```python
from build123d import *

# Parameters (mm, degrees)
F1_DEPTH = 3


with BuildPart() as f1:
    # F0 (on Top) → F1 (new body)
    with BuildSketch(Plane.XY):
        Polygon((-1.428907, -2.407704), (2.857814, 2.211777), (2.208733, 3.138307), (1.428907, 2.103039), (-2.857814, -2.516442), (-2.215881, -3.284665), align=None)
        Polygon((-2.857814, -4), (-2.215881, -3.284665), (-2.857814, -2.516442), align=None)
        Polygon((0.730746, -4), (-1.618143, -4), (-2.857814, -4), (-2.857814, -5), (2.005268, -5), (1.983487, -4), align=None)
        Polygon((1.633301, -2.505144), (1.983487, -4), (1.983487, -1.925149), align=None)
        Polygon((1.633301, -2.505144), (0.730746, -4), (1.983487, -4), align=None)
        Polygon((1.605074, 4), (2.857814, 4), (2.857814, 5), (-1.996555, 5), (-1.996555, 4), (-0.743815, 4), align=None)
        Polygon((-1.747311, 3.100817), (-1.996555, 4), (-1.996555, 2.877482), align=None)
        Polygon((-1.296617, 1.474879), (-1.747311, 3.100817), (-1.996555, 2.877482), (-1.996555, 1.474879), align=None)
        Polygon((-1.747311, 3.100817), (-0.743815, 4), (-1.996555, 4), align=None)
        Polygon((1.257835, -0.902368), (1.633301, -2.505144), (1.983487, -1.925149), (1.983487, -0.902368), align=None)
        Polygon((2.208733, 3.138307), (2.857814, 2.211777), (2.857814, 4), align=None)
        Polygon((-1.618143, -4), (-2.215881, -3.284665), (-2.857814, -4), align=None)
        Polygon((2.208733, 3.138307), (2.857814, 4), (1.605074, 4), align=None)
    extrude(amount=F1_DEPTH)


solid = f1.part
```
Geometry check sheet. Reference: the model listing, model coordinates, mm. A direction names the side the tool comes from. Give positions to 0.01 mm unless a question says otherwise; leave off trailing zeros. Loops run counter-clockwise (first coordinate to the right, second up) from the corner with the lowest first, then second, coordinate; pieces in that order, holes last. Notation, with made-up numbers: M -22,11.5 L 14,11.5 A10 cw 14,25.5 Z; hole C 41,76 d5. An arc over 180 degrees is marked long. Write item = value, one per line. Start each with the question number.
1. Tool access check on faces 1 (the face through (0, 5, 1)), 2 (the face through (1.983, -2, 1)), 3 (the face through (-1.52, 2.28, 1.48)). Record the directions out of +Z, -Z, +X, -X, +Y, -Y that give a thin tool (end or side, any length) a straight path to the whole face; none if there is none.
2. Draft check along X on faces 4 (the face through (-1.997, 3, 1)), 5 (the face through (0.684, -0.13, 1.479)), 6 (the face through (0, -5, 1)). Enter one of: +X half, -X half, draft (parallel to the pull), parting line (faces both ways), or undercut.
3. Section check B-B, the plane y = 2.75. Enter the section's corners in (x, z).
4. Section check A-A, the plane x = -0.85. Enter the section's corners in (y, z), plus the area to 3 significant figures.
5. Go/stop test with flat-tipped pins: P1, Ø0.9, axis at y = -2.5, z = 1, coming from the +X side; P2, Ø0.9, axis at y = 2.5, z = 1, coming from the -X side; P3, Ø1, axis at y = 1, z = 1, coming from the +X side. Record where each tip stops, or that it passes through.
6. Section check C-C, the plane z = 0.85. Enter the section's corners in (x, y), plus the area to 3 significant figures.
7. Thickness scan on probe 1 along Y at (x, z) = (0.55, 1.35); probe 2 along Y at (x, z) = (1.8, 1.1); probe 3 along X at (y, z) = (2, 1.5). Record the ranges inside material, lowest first.
8. Section check D-D, the plane x = 1.05. Enter the section's corners in (y, z).
Values follow:
q1.face_1 = +Z, -Z, +X, -X, +Y
q1.face_2 = +Z, -Z, +X
q1.face_3 = +Z, -Z
q2.face_4 = -X half
q2.face_5 = undercut
q2.face_6 = draft
q3.outline = M -2,0 L -1.65,0 L -1.65,3 L -2,3 Z; M 1.92,0 L 2.86,0 L 2.86,3 L 1.92,3 Z
q4.outline = M -5,0 L -4,0 L -4,3 L -5,3 Z; M -1.78,0 L -0.35,0 L -0.35,3 L -1.78,3 Z; M 3.9,0 L 5,0 L 5,3 L 3.9,3 Z
q4.area = 10.6 mm^2
q5.P1 = 1.98
q5.P2 = -2
q5.P3 = 2.2
q6.outline = M -2.86,-5 L 2.01,-5 L 1.98,-4 L 1.98,-0.9 L 1.26,-0.9 L 1.63,-2.51 L 0.73,-4 L -1.62,-4 L -2.22,-3.28 L -1.43,-2.41 L 2.86,2.21 L 2.86,5 L -2,5 L -2,1.47 L -1.3,1.47 L -1.75,3.1 L -0.74,4 L 1.61,4 L 2.21,3.14 L 1.43,2.1 L -2.86,-2.52 Z
q6.area = 22.7 mm^2
q7.probe_1 = -5 to -4, -0.28 to 1.16, 4 to 5
q7.probe_2 = -5 to -0.9, 1.07 to 2.6, 3.72 to 5
q7.probe_3 = -2 to -1.44, 1.33 to 2.66
q8.outline = M -5,0 L -3.47,0 L -3.47,3 L -5,3 Z; M 0.26,0 L 1.69,0 L 1.69,3 L 0.26,3 Z; M 4,0 L 5,0 L 5,3 L 4,3 Z
